Part model, mm, in its own coordinate system. Give positions to 0.01 mm unless a question says otherwise; leave off trailing zeros. Write each loop counter-clockwise with the first axis right and the second up, starting at its lowest first coordinate (ties: lowest second). Pieces come first, ordered by that corner, then holes. Notation, with made-up numbers: M 50.5,25.25 L 98.5,25.25 A16 ccw 98.5,48.25 Z; hole C 38,25.5 d5. An arc over 180 degrees is marked long. Use CSV: the item, a comma, the result in double quotes. Start each with the question number.
1. Band-saw the part on B-B, the plane y = 41. List the corners of the cut face in (x, z), then the cut area to 3 significant figures.
2. Drop flat-ended pins along their axis: pin 1 Ø1 at (x, z) = (15, 0.5) entering from -Y; pin 2 Ø3 at (x, y) = (12.5, 42.25) entering from +Z; pin 3 Ø1 at (x, z) = (14.5, 1.5) entering from +Y. Give the stop position or say it passes through.
3. Band-saw the part on C-C, the plane x = 20. List the corners of the cut face in (y, z), then the cut area to 3 significant figures.
4. Band-saw the part on D-D, the plane x = 1.5. List the corners of the cut face in (y, z), then the cut area to 3 significant figures.
5. Drill centre lines: line 1 along X through (y, z) = (4.5, 1.85); line 2 along Y through (x, z) = (12.5, 1.4); line 3 along X through (y, z) = (9, 0.8). Where is each one in solid material? Low to high. Write a range as from..to.
Autodesk Fusion 360 part; units mm, degrees
sketch "Sketch1" plane through (0, 0, 0) normal (0, 0, 1) x (1, 0, 0)
  line L0 (0, 0) -> (25, 0)
  line L1 (25, 0) -> (25, 55)
  line L2 (25, 55) -> (0, 55)
  line L3 (0, 55) -> (0, 0)
  dimension "d1" = 25
  dimension "d2" = 55
extrude "Extrude1" add sketch "Sketch1" along normal blind 2.5
sketch "Sketch2" plane through (0, 0, 0) normal (0, -1, 0) x (1, 0, 0)
  line L0 (0, 0) -> (25, 0)
  line L1 (25, 0) -> (25, 2.5)
  line L2 (25, 2.5) -> (0, 2.5)
  line L3 (0, 2.5) -> (0, 0)
  line L4 (0, 2.5) -> (4.5, 2.5)
  line L5 (4.5, 2.5) -> (4.5, 0)
  line L6 (4.5, 0) -> (0, 0)
  line L7 (0, 0) -> (0, 2.5)
  line L8 (25, 2.5) -> (20.5, 2.5)
  line L9 (20.5, 2.5) -> (20.5, 0)
  line L10 (20.5, 0) -> (25, 0)
  line L11 (25, 0) -> (25, 2.5)
  dimension "d5" = 4.5
  dimension "d6" = 4.5
extrude "Extrude2" cut sketch "Sketch2" against normal blind 3 contours L0 L2 L5 L9
sketch "Sketch3" plane through (0, 3, 0) normal (0, -1, 0) x (1, 0, 0)
  line L0 (4.5, 2.5) -> (4.5, 0)
  line L1 (4.5, 0) -> (20.5, 0)
  line L2 (20.5, 0) -> (20.5, 2.5)
  line L3 (20.5, 2.5) -> (4.5, 2.5)
  line L4 (10.75, 2.5) -> (14.25, 2.5)
  line L5 (14.25, 2.5) -> (14.25, 0)
  line L6 (14.25, 0) -> (10.75, 0)
  line L7 (10.75, 0) -> (10.75, 2.5)
  dimension "d9" = 3.5
  dimension "d10" = 6.25
extrude "Extrude3" cut sketch "Sketch3" against normal blind 4 contours L1 L3 L4 L5 L6 L7
sketch "Sketch4" plane through (0, 0, 2.5) normal (0, 0, 1) x (-1, 0, 0)
  line L0 (-10.75, -3) -> (-10.75, -7)
  line L1 (-10.75, -7) -> (-14.25, -7)
  line L2 (-14.25, -7) -> (-14.25, -3)
  line L3 (-14.25, -3) -> (-20.5, -3)
  line L4 (-20.5, -3) -> (-20.5, 0)
  line L5 (-20.5, 0) -> (-25, 0)
  line L6 (-25, 0) -> (-25, -55)
  line L7 (-25, -55) -> (0, -55)
  line L8 (0, -55) -> (0, 0)
  line L9 (0, 0) -> (-4.5, 0)
  line L10 (-4.5, 0) -> (-4.5, -3)
  line L11 (-4.5, -3) -> (-10.75, -3)
  line L12 (-9.5, -7) -> (-15.5, -7)
  line L13 (-15.5, -7) -> (-15.5, -10)
  line L14 (-15.5, -10) -> (-9.5, -10)
  line L15 (-9.5, -10) -> (-9.5, -7)
  dimension "d13" = 6
  dimension "d14" = 3
  dimension "d15" = 1.25
extrude "Extrude4" cut sketch "Sketch4" against normal blind 3 contours L1 L12 L13 L14 L15
sketch "Sketch5" plane through (0, 10, 0) normal (0, -1, 0) x (1, 0, 0)
  line L0 (9.5, 0) -> (15.5, 0)
  line L1 (15.5, 0) -> (15.5, 2.5)
  line L2 (15.5, 2.5) -> (9.5, 2.5)
  line L3 (9.5, 2.5) -> (9.5, 0)
  line L4 (10.75, 2.5) -> (14.25, 2.5)
  line L5 (14.25, 2.5) -> (14.25, 0)
  line L6 (14.25, 0) -> (10.75, 0)
  line L7 (10.75, 0) -> (10.75, 2.5)
  dimension "d18" = 3.5
  dimension "d19" = 2.5
  dimension "d20" = 1.25
extrude "Extrude5" cut sketch "Sketch5" against normal blind 2 contours L0 L2 L4 L5 L6 L7
sketch "Sketch6" plane through (0, 0, 2.5) normal (0, 0, 1) x (-1, 0, 0)
  line L0 (-10.75, -10) -> (-10.75, -12)
  line L1 (-10.75, -12) -> (-14.25, -12)
  line L2 (-14.25, -12) -> (-14.25, -10)
  line L3 (-14.25, -10) -> (-15.5, -10)
  line L4 (-15.5, -10) -> (-15.5, -7)
  line L5 (-15.5, -7) -> (-14.25, -7)
  line L6 (-14.25, -7) -> (-14.25, -3)
  line L7 (-14.25, -3) -> (-20.5, -3)
  line L8 (-20.5, -3) -> (-20.5, 0)
  line L9 (-20.5, 0) -> (-25, 0)
  line L10 (-25, 0) -> (-25, -55)
  line L11 (-25, -55) -> (0, -55)
  line L12 (0, -55) -> (0, 0)
  line L13 (0, 0) -> (-4.5, 0)
  line L14 (-4.5, 0) -> (-4.5, -3)
  line L15 (-4.5, -3) -> (-10.75, -3)
  line L16 (-10.75, -3) -> (-10.75, -7)
  line L17 (-10.75, -7) -> (-9.5, -7)
  line L18 (-9.5, -7) -> (-9.5, -10)
  line L19 (-9.5, -10) -> (-10.75, -10)
  circle A0 centre (-12.5, -42.25) radius 1.75
  dimension "d23" = 3.5
  dimension "d24" = 12.75
extrude "Extrude6" cut sketch "Sketch6" against normal blind 3 contours A0
fillet "Fillet1" radius 12.5 1 edges at (25, 55, 1.25)
fillet "Fillet2" radius 12.5 1 edges at (0, 55, 1.25)
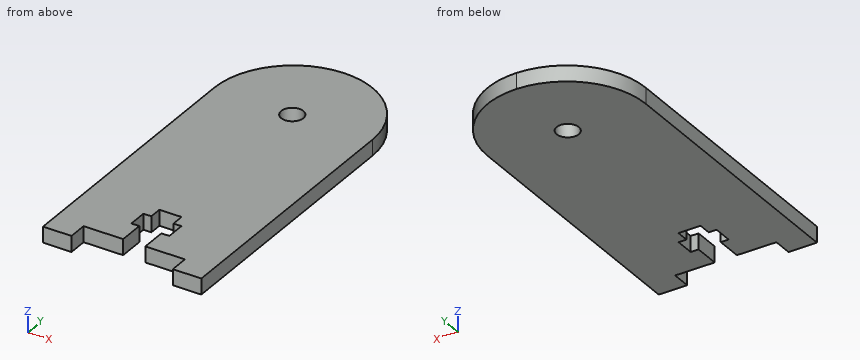
Output:
1,outline,"M 0,0 L 11.28,0 L 11.28,2.5 L 0,2.5 Z; M 13.72,0 L 25,0 L 25,2.5 L 13.72,2.5 Z"
1,area,"56.4 mm²"
2,pin 1,"stops at y = 3"
2,pin 2,"passes through"
2,pin 3,"stops at y = 54.91"
3,outline,"M 3,0 L 52.5,0 L 52.5,2.5 L 3,2.5 Z"
3,area,"124 mm²"
4,outline,"M 0,0 L 48.44,0 L 48.44,2.5 L 0,2.5 Z"
4,area,"121 mm²"
5,line 1,"x = 0..10.75, 14.25..25"
5,line 2,"y = 12..40.5, 44..55"
5,line 3,"x = 0..9.5, 15.5..25"
